For this review, take the finished solid that the model builds, in its own axes (mm). Face numbers are marked on the shaded views. A direction names the side the tool comes from. Round coordinates to 2 decimals unless told otherwise and drop trailing zeros. Loops run counter-clockwise (first coordinate to the right, second up) from the corner with the lowest first, then second, coordinate; pieces in that order, holes last.
```python
from build123d import *

# Parameters (mm, degrees)
SKETCH1_W                = 64
SKETCH1_H                = 307
SKETCH1_R                = 3
BOSS_EXTRUDE1_DEPTH      = 1
EDGE_FLANGE1_DEPTH       = 307
EDGE_FLANGE1_START       = 1
EDGE_FLANGE1_PROFILE_R   = 7.5
EDGE_FLANGE1_PROFILE_R_2 = 20
EDGE_FLANGE1_FLAT_DEPTH  = 1
EDGE_FLANGE2_DEPTH       = 260
EDGE_FLANGE2_START       = -1
EDGE_FLANGE2_PROFILE_R   = 3
EDGE_FLANGE2_FLAT_DEPTH  = 1
EDGE_FLANGE3_DEPTH       = 87
EDGE_FLANGE3_START       = -1
EDGE_FLANGE3_PROFILE_R   = 3
EDGE_FLANGE3_FLAT_DEPTH  = 1
EDGE_FLANGE4_DEPTH       = 307
EDGE_FLANGE4_START       = 1
EDGE_FLANGE4_PROFILE_R   = 4
EDGE_FLANGE4_FLAT_DEPTH  = 1
EDGE_FLANGE5_DEPTH       = 43.5
EDGE_FLANGE5_START       = 1
EDGE_FLANGE5_PROFILE_R   = 3
EDGE_FLANGE5_FLAT_DEPTH  = 1


# Sheet-metal steps are written as plain solids
with BuildPart() as part:
    # Sketch1 → Boss-Extrude1 (new body)
    with BuildSketch(Plane.XY):
        Rectangle(SKETCH1_W, SKETCH1_H)
        Circle(SKETCH1_R, mode=Mode.SUBTRACT)
        with Locations((0, 76.75)):
            Circle(SKETCH1_R, mode=Mode.SUBTRACT)
        with Locations((0, -76.75)):
            Circle(SKETCH1_R, mode=Mode.SUBTRACT)
    extrude(amount=BOSS_EXTRUDE1_DEPTH)

    # Edge-Flange1 bend section (across the edge) → Edge-Flange1 (add)
    with BuildSketch(Plane(origin=(-34, 153.5, 1), x_dir=(1, 0, 0), z_dir=(0, -1, 0))):
        with BuildLine():
            Line((-1, 2), (0, 2))
            ThreePointArc((0, 2), (0.585786438, 0.585786438), (2, 0))
            Line((2, 0), (2, -1))
            ThreePointArc((2, -1), (-0.121320344, -0.121320344), (-1, 2))
        make_face()
    extrude(amount=EDGE_FLANGE1_DEPTH)

    # Edge-Flange1 profile (on flange) → Edge-Flange1 flat (add)
    with BuildSketch(Plane(origin=(-34, 0, 1), x_dir=(0, -1, 0), z_dir=(-1, 0, 0)).offset(EDGE_FLANGE1_START)):
        with BuildLine():
            Line((-153.5, 89), (-153.5, 2))
            Line((-153.5, 2), (153.5, 2))
            Line((153.5, 2), (153.5, 20.25))
            Line((153.5, 20.25), (154.5, 20.25))
            ThreePointArc((154.5, 20.25), (155.207106781, 20.542893219), (155.5, 21.25))
            Line((155.5, 21.25), (155.5, 23.25))
            ThreePointArc((155.5, 23.25), (155.207106781, 23.957106781), (154.5, 24.25))
            Line((154.5, 24.25), (153.5, 24.25))
            Line((153.5, 24.25), (153.5, 89))
            ThreePointArc((153.5, 89), (130, 87), (106.5, 89))
            Line((106.5, 89), (-153.5, 89))
        make_face()
        with Locations((-133.5, 44.5)):
            Circle(EDGE_FLANGE1_PROFILE_R, mode=Mode.SUBTRACT)
        with Locations((0, 44.5)):
            Circle(EDGE_FLANGE1_PROFILE_R_2, mode=Mode.SUBTRACT)
        with Locations((-133.5, 66.75)):
            Circle(EDGE_FLANGE1_PROFILE_R, mode=Mode.SUBTRACT)
    extrude(amount=-EDGE_FLANGE1_FLAT_DEPTH)

    # Edge-Flange2 bend section (across the edge) → Edge-Flange2 (add)
    with BuildSketch(Plane(origin=(-35, -106.5, 92), x_dir=(0, 0, -1), z_dir=(0, 1, 0))):
        with BuildLine():
            Line((-1, 2), (0, 2))
            ThreePointArc((0, 2), (0.585786438, 0.585786438), (2, 0))
            Line((2, 0), (2, -1))
            ThreePointArc((2, -1), (-0.121320344, -0.121320344), (-1, 2))
        make_face()
    extrude(amount=EDGE_FLANGE2_DEPTH)

    # Edge-Flange2 profile (on flange) → Edge-Flange2 flat (add)
    with BuildSketch(Plane(origin=(-35, 0, 92), x_dir=(0, -1, 0), z_dir=(0, 0, -1)).offset(EDGE_FLANGE2_START)):
        with BuildLine():
            Line((-153.5, 2), (106.5, 2))
            Line((106.5, 2), (106.5, 18))
            ThreePointArc((106.5, 18), (105.914213562, 19.414213562), (104.5, 20))
            Line((104.5, 20), (-151.5, 20))
            ThreePointArc((-151.5, 20), (-152.914213562, 19.414213562), (-153.5, 18))
            Line((-153.5, 18), (-153.5, 2))
        make_face()
        with Locations((41.5, 10)):
            Circle(EDGE_FLANGE2_PROFILE_R, mode=Mode.SUBTRACT)
        with Locations((-88.5, 10)):
            Circle(EDGE_FLANGE2_PROFILE_R, mode=Mode.SUBTRACT)
    extrude(amount=EDGE_FLANGE2_FLAT_DEPTH)

    # Edge-Flange3 bend section (across the edge) → Edge-Flange3 (add)
    with BuildSketch(Plane(origin=(-35, 155.5, 90), x_dir=(0, -1, 0), z_dir=(0, 0, -1))):
        with BuildLine():
            Line((-1, 2), (0, 2))
            ThreePointArc((0, 2), (0.585786438, 0.585786438), (2, 0))
            Line((2, 0), (2, -1))
            ThreePointArc((2, -1), (-0.121320344, -0.121320344), (-1, 2))
        make_face()
    extrude(amount=EDGE_FLANGE3_DEPTH)

    # Edge-Flange3 profile (on flange) → Edge-Flange3 flat (add)
    with BuildSketch(Plane(origin=(-35, 155.5, 0), x_dir=(0, 0, 1), z_dir=(0, -1, 0)).offset(EDGE_FLANGE3_START)):
        with BuildLine():
            Line((3, 2), (90, 2))
            Line((90, 2), (90, 18))
            ThreePointArc((90, 18), (89.414213562, 19.414213562), (88, 20))
            Line((88, 20), (5, 20))
            ThreePointArc((5, 20), (3.585786438, 19.414213562), (3, 18))
            Line((3, 18), (3, 2))
        make_face()
        with Locations((24.75, 10)):
            Circle(EDGE_FLANGE3_PROFILE_R, mode=Mode.SUBTRACT)
        with Locations((68.25, 10)):
            Circle(EDGE_FLANGE3_PROFILE_R, mode=Mode.SUBTRACT)
    extrude(amount=EDGE_FLANGE3_FLAT_DEPTH)

    # Edge-Flange4 bend section (across the edge) → Edge-Flange4 (add)
    with BuildSketch(Plane(origin=(34, -153.5, 1), x_dir=(-1, 0, 0), z_dir=(0, 1, 0))):
        with BuildLine():
            Line((-1, 2), (0, 2))
            ThreePointArc((0, 2), (0.585786438, 0.585786438), (2, 0))
            Line((2, 0), (2, -1))
            ThreePointArc((2, -1), (-0.121320344, -0.121320344), (-1, 2))
        make_face()
    extrude(amount=EDGE_FLANGE4_DEPTH)

    # Edge-Flange4 profile (on flange) → Edge-Flange4 flat (add)
    with BuildSketch(Plane(origin=(34, 0, 1), x_dir=(0, 1, 0), z_dir=(1, 0, 0)).offset(EDGE_FLANGE4_START)):
        with BuildLine():
            ThreePointArc((-155.5, 21.25), (-155.207106781, 20.542893219), (-154.5, 20.25))
            Line((-154.5, 20.25), (-153.5, 20.25))
            Line((-153.5, 20.25), (-153.5, 2))
            Line((-153.5, 2), (153.5, 2))
            Line((153.5, 2), (153.5, 45.5))
            Line((153.5, 45.5), (-153.5, 45.5))
            Line((-153.5, 45.5), (-153.5, 24.25))
            Line((-153.5, 24.25), (-154.5, 24.25))
            ThreePointArc((-154.5, 24.25), (-155.207106781, 23.957106781), (-155.5, 23.25))
            Line((-155.5, 23.25), (-155.5, 21.25))
        make_face()
        with Locations((-76.75, 22.75)):
            Circle(EDGE_FLANGE4_PROFILE_R, mode=Mode.SUBTRACT)
        with Locations((76.75, 22.75)):
            Circle(EDGE_FLANGE4_PROFILE_R, mode=Mode.SUBTRACT)
    extrude(amount=-EDGE_FLANGE4_FLAT_DEPTH)

    # Edge-Flange5 bend section (across the edge) → Edge-Flange5 (add)
    with BuildSketch(Plane(origin=(35, 155.5, 3), x_dir=(0, -1, 0), z_dir=(0, 0, 1))):
        with BuildLine():
            Line((-1, 2), (0, 2))
            ThreePointArc((0, 2), (0.585786438, 0.585786438), (2, 0))
            Line((2, 0), (2, -1))
            ThreePointArc((2, -1), (-0.121320344, -0.121320344), (-1, 2))
        make_face()
    extrude(amount=EDGE_FLANGE5_DEPTH)

    # Edge-Flange5 profile (on flange) → Edge-Flange5 flat (add)
    with BuildSketch(Plane(origin=(35, 155.5, 0), x_dir=(0, 0, 1), z_dir=(0, 1, 0)).offset(EDGE_FLANGE5_START)):
        with BuildLine():
            ThreePointArc((5, 20), (3.585786438, 19.414213562), (3, 18))
            Line((3, 18), (3, 2))
            Line((3, 2), (46.5, 2))
            Line((46.5, 2), (46.5, 18))
            ThreePointArc((46.5, 18), (45.914213562, 19.414213562), (44.5, 20))
            Line((44.5, 20), (5, 20))
        make_face()
        with Locations((24.75, 10)):
            Circle(EDGE_FLANGE5_PROFILE_R, mode=Mode.SUBTRACT)
    extrude(amount=-EDGE_FLANGE5_FLAT_DEPTH)


solid = part.part
```
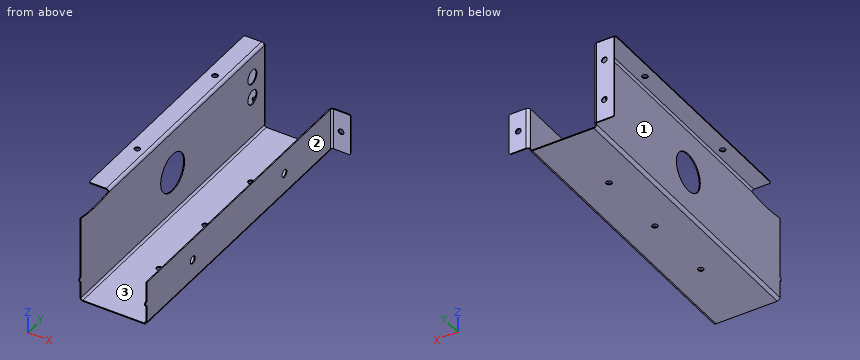
(1) Add section D-D (x = 45). Give the boundary of the cut face in (y, z).
(2) Insertion check: pin 1 Ø1 at (y, z) = (107, 43) entering from +X; pin 2 Ø0.9 at (x, y) = (-47.5, 154.5) entering from -Z; pin 3 Ø5.5 at (x, z) = (48, 30) entering from -Y; pin 4 Ø2 at (x, y) = (18.5, -110.5) entering from -Z. Each pin has a flat end and moves straight along its axis. Give the tip position at first contact, or say it passes through.
(3) For L1, parallel to Y at x = 0, z = 0.65; L2, parallel to X at y = -105.5, z = 46; L3, parallel to Y at x = -39, z = 50.5, list the stretches that pass through material, from the lowest coordinate up.
(4) For the marked faces 1, 2 and 3, list the 3-axis set-ups (+Z, -Z, +X, -X, +Y, -Y) from which the entire face can be reached by the end or side of a thin tool; tool diameter is ignored.
(5) Add section A-A (z = 9.5). Give the boundary of the cut face in (x, y), plus the area to 3 significant figures.
(6) Add section B-B (x = 0). Give the boundary of the cut face in (y, z).
(7) Add section C-C (y = 76.75). Give the boundary of the cut face in (x, z), plus the area to 3 significant figures.
Outcome:
1. outline: (155.5, 3) - (156.5, 3) - (156.5, 21.75) - (155.5, 21.75) - close; (155.5, 27.75) - (156.5, 27.75) - (156.5, 46.5) - (155.5, 46.5) - close
2. pin 1: stops at x = 35
2. pin 2: passes through
2. pin 3: stops at y = 155.5
2. pin 4: stops at z = 0
3. L1: y = -153.5 to -79.75, -73.75 to -3, 3 to 73.75, 79.75 to 153.5
3. L2: x = -35 to -34, 34 to 35
3. L3: y = 155.5 to 156.5
4. face 1: -Z, -X, -Y
4. face 2: +Z, -Z, +X, -Y
4. face 3: +Z, +Y, -Y
5. outline: (-55, 155.5) - (-37, 155.5) arc R2 cw to (-35, 153.5) - (-35, -153.5) - (-34, -153.5) - (-34, 153.5) arc R3 ccw to (-37, 156.5) - (-55, 156.5) - close; (34, -153.5) - (35, -153.5) - (35, 153.5) arc R2 cw to (37, 155.5) - (55, 155.5) - (55, 156.5) - (37, 156.5) arc R3 ccw to (34, 153.5) - close
5. area: 658 mm2
6. outline: (-153.5, 0) - (-79.75, 0) - (-79.75, 1) - (-153.5, 1) - close; (-73.75, 0) - (-3, 0) - (-3, 1) - (-73.75, 1) - close; (3, 0) - (73.75, 0) - (73.75, 1) - (3, 1) - close; (79.75, 0) - (153.5, 0) - (153.5, 1) - (79.75, 1) - close
7. outline: (-55, 92) - (-37, 92) arc R2 cw to (-35, 90) - (-35, 3) arc R3 ccw to (-32, 0) - (-3, 0) - (-3, 1) - (-32, 1) arc R2 cw to (-34, 3) - (-34, 90) arc R3 ccw to (-37, 93) - (-55, 93) - close; (3, 0) - (32, 0) arc R3 ccw to (35, 3) - (35, 19.75) - (34, 19.75) - (34, 3) arc R2 cw to (32, 1) - (3, 1) - close; (34, 27.75) - (35, 27.75) - (35, 46.5) - (34, 46.5) - close
7. area: 210 mm2
